Input: dimensioned drawing with shaded views. Units: mm. Origin: part minimum x, y, z. Round coordinates to 2 decimals unless told otherwise and drop trailing zeros. Order: outer loops, then holes, each group sorted by start corner. A loop starts at its lowest first (then second) coordinate and runs counter-clockwise, first axis right, second up. Notation, with made-up numbers: M -19,25 L 23,25 A12 cw 23,40 Z; hole C -38.5,42 d10. An arc over 180 degrees is marked long. Use CSV: the item, a comma, the result in double quotes. Start each with the question number.
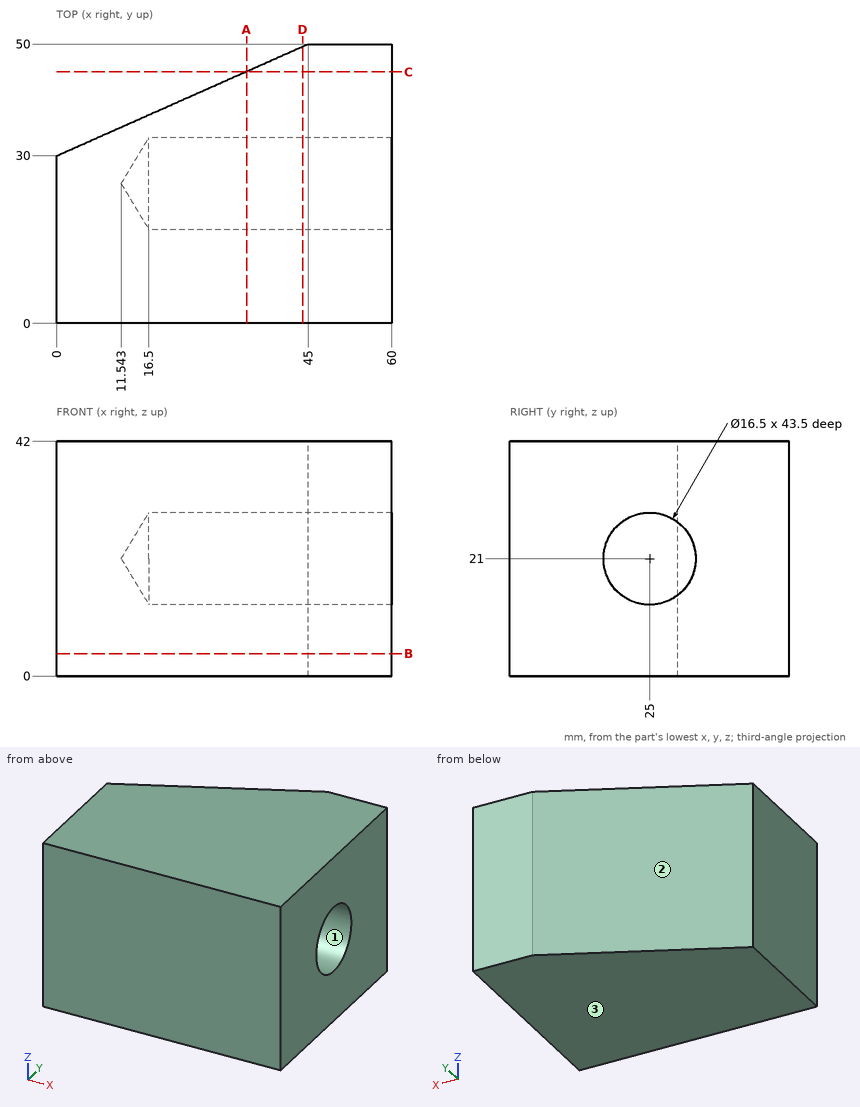
(1) Section C-C on y = 45. Return loops of the section in (x, z).
(2) Section B-B on z = 4. Return loops of the section in (x, y), plus the area to 3 significant figures.
(3) Contact query for flat-ended pins moving along their axis: P1, Ø3, axis at y = 38.5, z = 24, coming from the -X side; P2, Ø1.5, axis at y = 44, z = 7.5, coming from the -X side; P3, Ø5, axis at x = 24.5, z = 17, coming from the +Y side. Output: stop coordinate, or through.
(4) Draft query along Z for the marked faces 1, 2 and 3. Return one class per face: pulls with the +Z half, pulls with the -Z half, needs draft (parallel to the pull), parting line crosses it, or undercut.
(5) Section D-D on x = 44. Return loops of the section in (y, z).
(6) Line query: line 1 along Z through (x, y) = (36, 25); line 2 along Y through (x, z) = (50, 21); line 3 along Y through (x, z) = (42.5, 21). Output: solid intervals per line, ascending.
(7) Section A-A on x = 34. Return loops of the section in (y, z), plus the area to 3 significant figures.
Results below:
1,outline,"M 33.75,0 L 60,0 L 60,42 L 33.75,42 Z"
2,outline,"M 0,0 L 60,0 L 60,50 L 45,50 L 0,30 Z"
2,area,"2,550 mm2"
3,P1,"stops at x = 15.75"
3,P2,"stops at x = 29.81"
3,P3,"stops at y = 42"
4,face 1,"undercut"
4,face 2,"needs draft"
4,face 3,"pulls with the -Z half"
5,outline,"M 0,0 L 49.56,0 L 49.56,42 L 0,42 Z; hole C 25,21 d16.5"
6,line 1,"z = 0 to 12.75, 29.25 to 42"
6,line 2,"y = 0 to 16.75, 33.25 to 50"
6,line 3,"y = 0 to 16.75, 33.25 to 48.89"
7,outline,"M 0,0 L 45.11,0 L 45.11,42 L 0,42 Z; hole C 25,21 d16.5"
7,area,"1,680 mm2"
